Check sheet for the drawn part. Datum: minimum x, y, z corner. Units: mm. A direction names the side the tool comes from. Round coordinates to 2 decimals unless told otherwise and drop trailing zeros. Loops run counter-clockwise (first coordinate to the right, second up) from the corner with the lowest first, then second, coordinate; pieces in that order, holes last. Notation, with made-up numbers: (41, 37) -> (89, 37) arc R5 cw to (89, 46) -> close; hole circle Ø2 at (-0.5, 1). An arc over 180 degrees is marked (long way). Return JSON: item names as keys, results as strings.
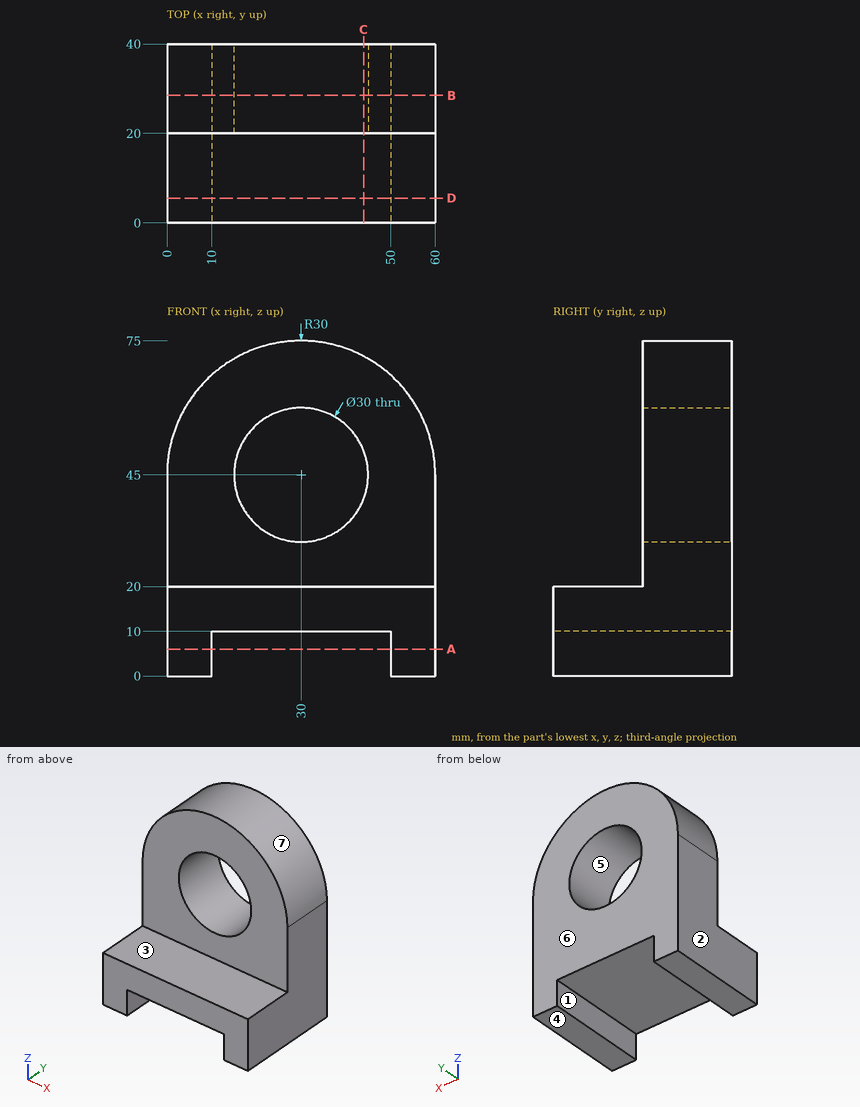
Q1. Tool access check on the marked faces 1, 2 and 3. Record the directions out of +Z, -Z, +X, -X, +Y, -Y that give a thin tool (end or side, any length) a straight path to the whole face; none if there is none.
Results list:
{"face 1": "-Z, +Y, -Y", "face 2": "+Z, -Z, -X, +Y, -Y", "face 3": "+Z, +X, -X, -Y"}
Q2. Section check A-A (z = 6). Record the boundary of the cut face in (x, y), then the cut area to 3 significant figures.
Results list:
{"outline": "(0, 0) -> (10, 0) -> (10, 40) -> (0, 40) -> close; (50, 0) -> (60, 0) -> (60, 40) -> (50, 40) -> close", "area": "800 mm^2"}
Q3. Draft check along Z on the marked faces 4, 5, 6 and 7. Enter one of: released by +Z, released by -Z, zero draft, split by the parting line, or undercut.
Results list:
{"face 4": "released by -Z", "face 5": "undercut", "face 6": "zero draft", "face 7": "released by +Z"}
Q4. Section check D-D (y = 5.5). Record the boundary of the cut face in (x, z).
Results list:
{"outline": "(0, 0) -> (10, 0) -> (10, 10) -> (50, 10) -> (50, 0) -> (60, 0) -> (60, 20) -> (0, 20) -> close"}
Q5. Material ranges on line 1 (Z direction, x = 30, y = 28.5); line 2 (Y direction, x = 19.5, z = 30); line 3 (Z direction, x = 28, y = 5), recorded low to high.
Results list:
{"line 1": "10 to 30, 60 to 75", "line 2": "20 to 40", "line 3": "10 to 20"}
Q6. Section check C-C (x = 44). Record the boundary of the cut face in (y, z).
Results list:
{"outline": "(0, 10) -> (40, 10) -> (40, 39.61) -> (20, 39.61) -> (20, 20) -> (0, 20) -> close; (20, 50.39) -> (40, 50.39) -> (40, 71.53) -> (20, 71.53) -> close"}
Q7. Section check B-B (y = 28.5). Record the boundary of the cut face in (x, z).
Results list:
{"outline": "(0, 0) -> (10, 0) -> (10, 10) -> (50, 10) -> (50, 0) -> (60, 0) -> (60, 45) arc R30 ccw to (0, 45) -> close; hole circle Ø30 at (30, 45)"}
Q8. Go/stop test with flat-tipped pins: pin 1 (24 mm diameter, centred on x = 30, z = 45, fed in from -Y); pin 2 (3 mm diameter, centred on x = 26.5, y = 9.5, fed in from -Z); pin 3 (6 mm diameter, centred on x = 33, y = 11.5, fed in from +Z); pin 4 (3 mm diameter, centred on y = 16.5, z = 3, fed in from -X). Record where each tip stops, or that it passes through.
Results list:
{"pin 1": "through", "pin 2": "z = 10", "pin 3": "z = 20", "pin 4": "x = 0"}
